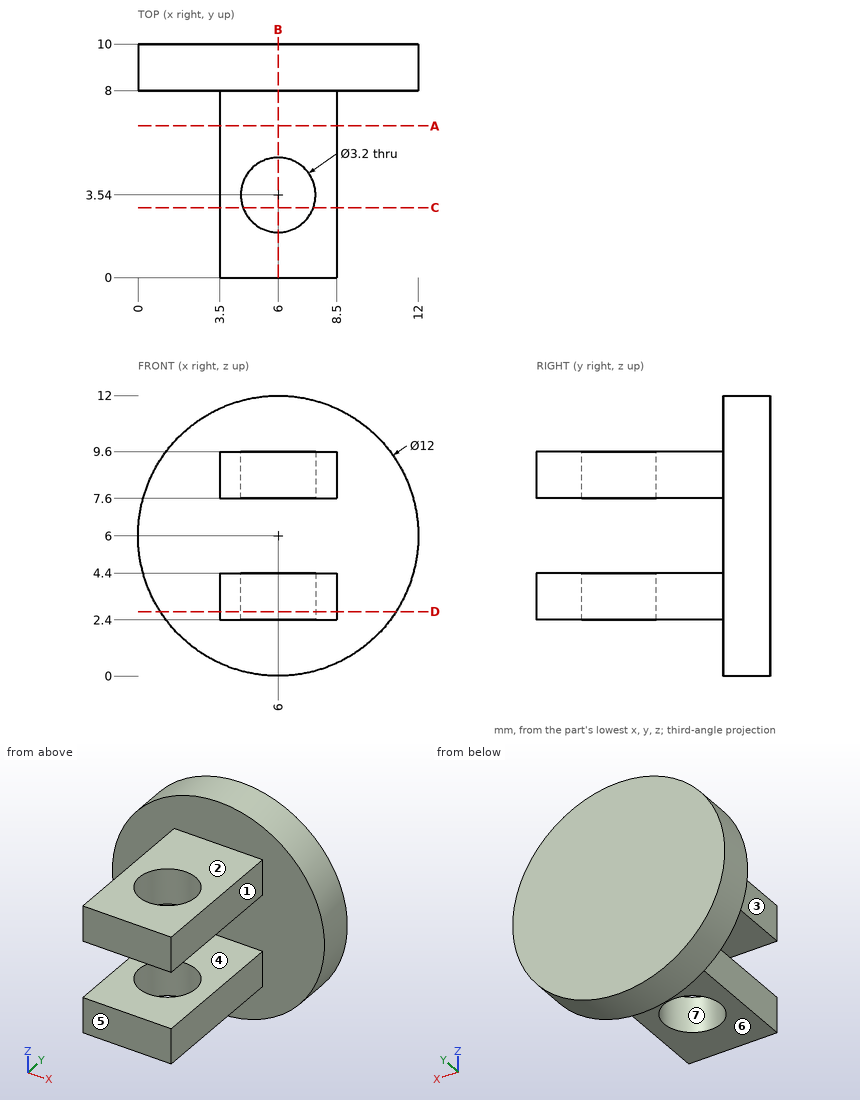
For this review, use the dimensioned drawing (mm, ordinates from the lowest corner) and the shaded views. A direction names the side the tool comes from. Round coordinates to 2 decimals unless told otherwise and drop trailing zeros. Loops run counter-clockwise (first coordinate to the right, second up) from the corner with the lowest first, then second, coordinate; pieces in that order, holes last. Notation, with made-up numbers: (30.5, -26) -> (67.5, -26) arc R31 cw to (67.5, 5) -> close; hole circle Ø8 at (52, 88.5). An arc over 180 degrees is marked (long way). Write item = value, one per line. Start each with the question number.
Item 1: Insertion check: pin 1 (1.5 mm diameter, centred on x = 5.5, y = 3.5, fed in from +Z); pin 2 (4 mm diameter, centred on x = 7, y = 5.5, fed in from +Z); pin 3 (1.6 mm diameter, centred on y = 3, z = 3, fed in from -X); pin 4 (0.6 mm diameter, centred on y = 2.5, z = 3.5, fed in from +X). Each pin has a flat end and moves straight along its axis. Give the tip position at first contact, or say it passes through.
Item 2: Take a section at A-A on y = 6.5. Give the boundary of the cut face in (x, z).
Item 3: Take a section at B-B on x = 6. Give the boundary of the cut face in (y, z).
Item 4: For the marked faces 1, 2, 3 and 4, list the 3-axis set-ups (+Z, -Z, +X, -X, +Y, -Y) from which the entire face can be reached by the end or side of a thin tool; tool diameter is ignored.
Item 5: Mouldability with a two-part tool opening along Y and no side actions: class the marked faces 5, 6 and 7 as released by +Y, released by -Y, zero draft, split by the parting line, or undercut.
Item 6: Take a section at D-D on z = 2.75. Give the boundary of the cut face in (x, y).
Item 7: To check wall thickness, follow L1, parallel to Z at x = 6, y = 7.25; L2, parallel to Y at x = 6, z = 9.1; L3, parallel to X at y = 4.75, z = 9.5. State the ranges of each line that lie inside material, in increasing order.
Item 8: Take a section at C-C on y = 3. Give the boundary of the cut face in (x, z), plus the area to 3 significant figures.
Result:
q1.pin_1 = through
q1.pin_2 = 9.6
q1.pin_3 = 3.5
q1.pin_4 = 8.5
q2.outline = (3.5, 2.4) -> (8.5, 2.4) -> (8.5, 4.4) -> (3.5, 4.4) -> close; (3.5, 7.6) -> (8.5, 7.6) -> (8.5, 9.6) -> (3.5, 9.6) -> close
q3.outline = (0, 2.4) -> (1.94, 2.4) -> (1.94, 4.4) -> (0, 4.4) -> close; (0, 7.6) -> (1.94, 7.6) -> (1.94, 9.6) -> (0, 9.6) -> close; (5.14, 2.4) -> (8, 2.4) -> (8, 0) -> (10, 0) -> (10, 12) -> (8, 12) -> (8, 9.6) -> (5.14, 9.6) -> (5.14, 7.6) -> (8, 7.6) -> (8, 4.4) -> (5.14, 4.4) -> close
q4.face_1 = +Z, -Z, +X, -Y
q4.face_2 = +Z, +X, -X, -Y
q4.face_3 = +Z, -Z, -X, -Y
q4.face_4 = +X, -X, -Y
q5.face_5 = released by -Y
q5.face_6 = zero draft
q5.face_7 = undercut
q6.outline = (0.96, 8) -> (3.5, 8) -> (3.5, 0) -> (8.5, 0) -> (8.5, 8) -> (11.04, 8) -> (11.04, 10) -> (0.96, 10) -> close; hole circle Ø3.2 at (6, 3.54)
q7.L1 = 2.4 to 4.4, 7.6 to 9.6
q7.L2 = 0 to 1.94, 5.14 to 10
q7.L3 = 3.5 to 4.95, 7.05 to 8.5
q8.outline = (3.5, 2.4) -> (4.49, 2.4) -> (4.49, 4.4) -> (3.5, 4.4) -> close; (3.5, 7.6) -> (4.49, 7.6) -> (4.49, 9.6) -> (3.5, 9.6) -> close; (7.51, 2.4) -> (8.5, 2.4) -> (8.5, 4.4) -> (7.51, 4.4) -> close; (7.51, 7.6) -> (8.5, 7.6) -> (8.5, 9.6) -> (7.51, 9.6) -> close
q8.area = 7.95 mm²
